Autodesk Inventor part; units mm, degrees
ref_plane "Work Plane1" through (0, 2.4, 0) normal (0, 1, 0) x (1, 0, 0)
ref_plane "YZ Plane" through (0, 0, 0) normal (1, 0, 0) x (0, 1, 0)
ref_plane "XZ Plane" through (0, 0, 0) normal (0, 1, 0) x (-1, 0, 0)
sketch "Sketch1" plane through (0, 0, 0) normal (0, 1, 0) x (-1, 0, 0)
  line L0 (2.95, 6.425) -> (-2.95, 6.425)
  line L1 (-2.95, 6.425) -> (-2.95, -6.425)
  line L2 (-2.95, -6.425) -> (2.95, -6.425)
  line L3 (2.95, -6.425) -> (2.95, 6.425)
  line L4 (4.13, 0) -> (-4.13, 0) construction
  line L5 (0, -8.995) -> (0, 8.995) construction
  point P0 (0, 0)
  dimension "d0" = 5.9
  dimension "d1" = 12.85
extrude "Extrusion1" add sketch "Sketch1" along normal blind 6.6
sketch "Sketch2" plane through (2.95, 0, 6.425) normal (1, 0, 0) x (0, 0, -1)
  circle A0 centre (3.15, 1.5) radius 0.7
  circle A1 centre (9.65, 1.5) radius 0.5
  line L0 (0, 0) -> (0, 6.6)
  line L1 (0, 0) -> (12.85, 0)
  point P0 (6.425, 0)
  dimension "d4" = 1.4
  dimension "d5" = 1
  dimension "d6" = 3.15
  dimension "d7" = 6.5
  dimension "d8" = 1.5
extrude "Extrusion2" cut sketch "Sketch2" against normal through all
sketch "Sketch3" plane through (0, 0, 0) normal (1, 0, 0) x (0, 1, 0)
  line L0 (6.6, -6.425) -> (6.6, 6.425)
  circle A0 centre (6.6, 1.975) radius 0.575
  circle A1 centre (1.5, -3.225) radius 0.5
  point P0 (0, 0)
  point P1 (6.6, 2.55)
  point P2 (6.6, 1.4)
  dimension "d11" = 1.15
  dimension "d12" = 5.2
extrude "Extrusion3" add sketch "Sketch3" along normal mid plane 2.75 contours L0 A0 picked at (6.6832, 2.1477)
sketch "Sketch4" plane through (0, 0, 0) normal (1, 0, 0) x (0, 1, 0)
  line L0 (0, 6.425) -> (0, -6.425)
  line L1 (0, 0.45) -> (-2.75, 0.45)
  line L2 (0, -0.45) -> (-2.75, -0.45)
  arc A0 (-2.75, 0.45) -> (-2.75, -0.45) centre (-2.75, 0) ccw
  line L3 (-5.275, 0) -> (9.25, 0) construction
  point P0 (0, 0)
  point P1 (-3.2, 0)
  dimension "d15" = 3.2
  dimension "d16" = 0.9
extrude "Extrusion4" add sketch "Sketch4" along normal mid plane 0.4
pattern_linear "Rectangular Pattern1" count 2 spacing 5.08 along (0, 0, -1) count 2 spacing 5.08 along (0, 0, 1) of "Extrusion4"
ref_plane "Work Plane1" through (0, 2.4, 0) normal (0, 1, 0) x (1, 0, 0)
split_face "Split1"
properties part number "Kailh_GM_8.0_switch"
Input: part model. Units: mm. Frame: model coordinates. A direction names the side the tool comes from. Round coordinates to 2 decimals unless told otherwise and drop trailing zeros. Order: outer loops, then holes, each group sorted by start corner. A loop starts at its lowest first (then second) coordinate and runs counter-clockwise, first axis right, second up. Notation, with made-up numbers: (-24, -8) - (-8, -8) arc R19 ccw to (-8, 26) - close; hole circle Ø5 at (42, 33). An arc over 180 degrees is marked (long way). Use a Markdown table: item, result.
1. Section A-A on y = 1.5. Return the cut outline in (x, z) (3 decimals), then the cut area to 3 significant figures.
Evaluation:
| item | result |
|---|---|
| outline | (-2.95, -6.425) - (2.95, -6.425) - (2.95, -3.725) - (-2.95, -3.725) - close; (-2.95, -2.725) - (2.95, -2.725) - (2.95, 2.575) - (-2.95, 2.575) - close; (-2.95, 3.975) - (2.95, 3.975) - (2.95, 6.425) - (-2.95, 6.425) - close |
| area | 61.7 mm^2 |
2. Section D-D on z = 3. Return the cut outline in (x, y).
Evaluation:
| item | result |
|---|---|
| outline | (-2.95, 0) - (2.95, 0) - (2.95, 0.86) - (-2.95, 0.86) - close; (-2.95, 2.14) - (2.95, 2.14) - (2.95, 6.6) - (-2.95, 6.6) - close |
3. Section C-C on z = 5.08. Return the cut outline in (x, y).
Evaluation:
| item | result |
|---|---|
| outline | (-2.95, 0) - (-0.2, 0) - (-0.2, -3.2) - (0.2, -3.2) - (0.2, 0) - (2.95, 0) - (2.95, 6.6) - (-2.95, 6.6) - close |
4. Material intervals for probe 1 along Y at (x, z) = (-0.55, -0.75); probe 2 along Y at (x, z) = (-0.3, 1.5), sorted ascending.
Evaluation:
| item | result |
|---|---|
| probe 1 | 0 to 6.6 |
| probe 2 | 0 to 6.92 |
5. First-contact query: pin 1 (2 mm diameter, centred on x = 1.5, z = -4.5, fed in from -Y); pin 2 (0.7 mm diameter, centred on y = -2, z = 5, fed in from -X); pin 3 (0.7 mm diameter, centred on y = -1, z = 5, fed in from +X). Flat tips, straight axial feed; report the tip coordinate or a pass-through.
Evaluation:
| item | result |
|---|---|
| pin 1 | y = 0 |
| pin 2 | x = -0.2 |
| pin 3 | x = 0.2 |
6. Mould query, pull axis Y, two halves, no side actions, for faces 4 (the face through (-0.2, -2, -5)), 5 (the face through (0.04, 1.65, -3.7)), 6 (the face through (0, 6.6, 0)). Classes: +Y half, -Y half, draft (parallel to the pull), parting line (faces both ways), or undercut.
Evaluation:
| item | result |
|---|---|
| face 4 | draft |
| face 5 | undercut |
| face 6 | +Y half |
7. Access query for faces 1 (the face through (-0.2, -2, 0)), 2 (the face through (-2.95, 3, 0)), 3 (the face through (0.2, -2, 0)). Directions: +Z, -Z, +X, -X, +Y, -Y. A direction counts if a zero-diameter tool reaches every point of the face in a straight line with its end or side. Return the directions, or none.
Evaluation:
| item | result |
|---|---|
| face 1 | +Z, -Z, -X, -Y |
| face 2 | +Z, -Z, -X, +Y, -Y |
| face 3 | +Z, -Z, +X, -Y |
8. Section B-B on x = 1. Return the cut outline in (y, z) (3 decimals).
Evaluation:
| item | result |
|---|---|
| outline | (0, -6.425) - (6.6, -6.425) - (6.6, 1.4) arc R0.575 ccw to (6.6, 2.55) - (6.6, 6.425) - (0, 6.425) - close; hole circle Ø1.4 at (1.5, 3.275); hole circle Ø1 at (1.5, -3.225) |
